The drawing under review shows one solid part. Ordinate dimensions are in mm from its lowest x, y, z. Coordinates: 2 decimals unless noted, no trailing zeros. Order: outer loops, then holes, each group sorted by start corner. A loop starts at its lowest first (then second) coordinate and runs counter-clockwise, first axis right, second up. Notation, with made-up numbers: (10.5, -22.75) -> (58.5, -22.75) arc R22 ccw to (58.5, 2.25) -> close; hole circle Ø2 at (-26, -15.75). An arc over 180 degrees is marked (long way). Use one line per item in the form item = value.
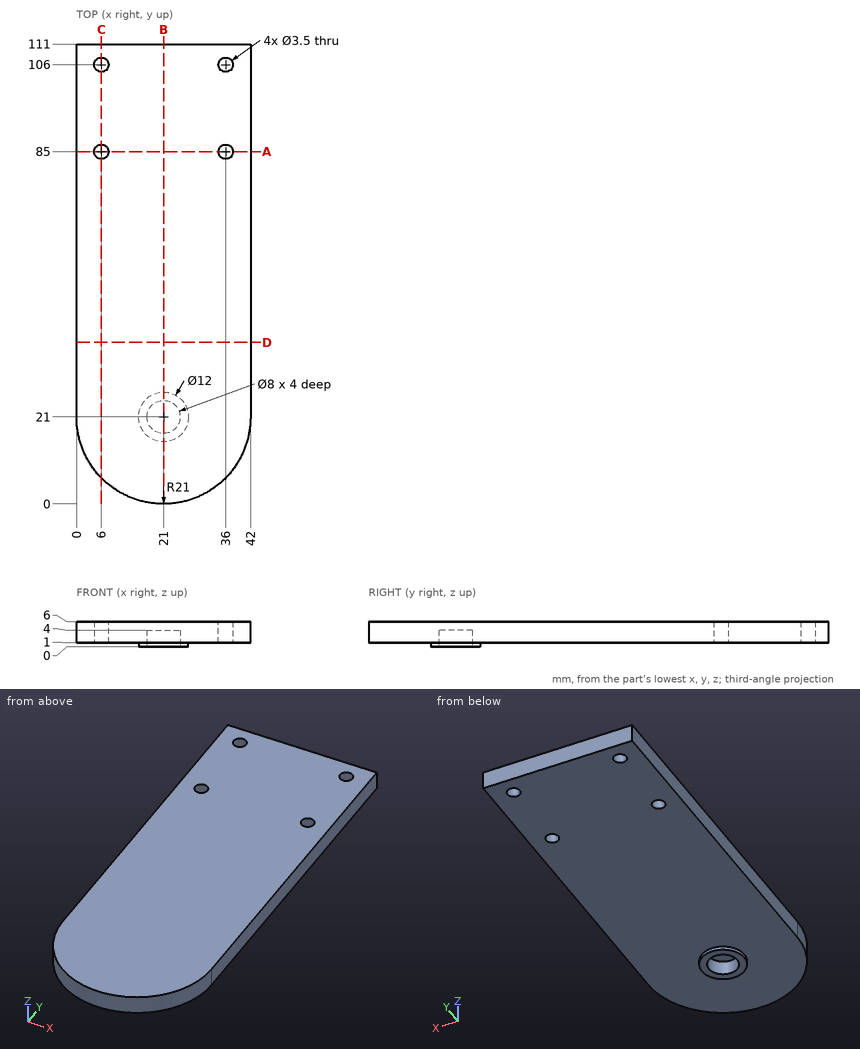
Item 1: To check wall thickness, follow L1, parallel to X at y = 106, z = 4.5; L2, parallel to Y at x = 6, z = 2.7; L3, parallel to Z at x = 15, y = 24. State the ranges of each line that lie inside material, in increasing order. Write a range as from..to.
Results found:
L1 = 0..4.25, 7.75..34.25, 37.75..42
L2 = 6.3..83.25, 86.75..104.25, 107.75..111
L3 = 1..6
Item 2: We need section B-B (x = 21). Write out the cut boundary in (y, z).
Results found:
outline = (0, 1) -> (15, 1) -> (15, 0) -> (17, 0) -> (17, 4) -> (25, 4) -> (25, 0) -> (27, 0) -> (27, 1) -> (111, 1) -> (111, 6) -> (0, 6) -> close
Item 3: We need section D-D (y = 39). Write out the cut boundary in (x, z), plus the area to 3 significant figures.
Results found:
outline = (0, 1) -> (42, 1) -> (42, 6) -> (0, 6) -> close
area = 210 mm²
Item 4: We need section A-A (y = 85). Write out the cut boundary in (x, z), plus the area to 3 significant figures.
Results found:
outline = (0, 1) -> (4.25, 1) -> (4.25, 6) -> (0, 6) -> close; (7.75, 1) -> (34.25, 1) -> (34.25, 6) -> (7.75, 6) -> close; (37.75, 1) -> (42, 1) -> (42, 6) -> (37.75, 6) -> close
area = 175 mm²
Item 5: Clearance check with flat-ended pins moving along their axes: pin 1 (2 mm diameter, centred on x = 9, z = 4.5, fed in from -Y); pin 2 (4 mm diameter, centred on x = 36, y = 85, fed in from -Z); pin 3 (1 mm diameter, centred on x = 15.5, z = 4, fed in from -Y). State where each tip first meets the part, or that it passes through.
Results found:
pin_1 = 3.11
pin_2 = 1
pin_3 = 0.6
Item 6: We need section C-C (x = 6). Write out the cut boundary in (y, z).
Results found:
outline = (6.3, 1) -> (83.25, 1) -> (83.25, 6) -> (6.3, 6) -> close; (86.75, 1) -> (104.25, 1) -> (104.25, 6) -> (86.75, 6) -> close; (107.75, 1) -> (111, 1) -> (111, 6) -> (107.75, 6) -> close
